For this review, take the finished solid that the model builds, in its own axes (mm). A direction names the side the tool comes from. Coordinates: 2 decimals unless noted, no trailing zeros. Order: outer loops, then holes, each group sorted by start corner. A loop starts at its lowest first (then second) coordinate and runs counter-clockwise, first axis right, second up.
from build123d import *

# Parameters (mm, degrees)
F1_DEPTH = 25
F2_R     = 8
F3_DEPTH = 37.501


with BuildPart() as f1:
    # F0 (on Front) → F1 (new body)
    with BuildSketch(Plane.XZ):
        with BuildLine():
            Line((-51.7705098312, 2.5), (-22.360679775, 2.5))
            ThreePointArc((-22.360679775, 2.5), (-20.5395959064, 9.1855865354), (-16.7705098312, 15))
            Line((-16.7705098312, 15), (-51.7705098312, 15))
            Line((-51.7705098312, 15), (-51.7705098312, 2.5))
        make_face()
        with BuildLine():
            ThreePointArc((-16.7705098312, -15), (-20.5395959064, -9.1855865354), (-22.360679775, -2.5))
            Line((-22.360679775, -2.5), (-51.7705098312, -2.5))
            Line((-51.7705098312, -2.5), (-51.7705098312, -15))
            Line((-51.7705098312, -15), (-16.7705098312, -15))
        make_face()
        with BuildLine():
            ThreePointArc((-14.7901994577, 2.5), (1.2543939042, 14.9474578418), (15, 0))
            ThreePointArc((15, 0), (1.2543939042, -14.9474578418), (-14.7901994577, -2.5))
            Line((-14.7901994577, -2.5), (-22.360679775, -2.5))
            ThreePointArc((-22.360679775, -2.5), (-20.5395959064, -9.1855865354), (-16.7705098312, -15))
            ThreePointArc((-16.7705098312, -15), (8.0284970199, -21.0188780767), (22.5, 0))
            ThreePointArc((22.5, 0), (8.0284970199, 21.0188780767), (-16.7705098312, 15))
            ThreePointArc((-16.7705098312, 15), (-20.5395959064, 9.1855865354), (-22.360679775, 2.5))
            Line((-22.360679775, 2.5), (-14.7901994577, 2.5))
        make_face()
    extrude(amount=F1_DEPTH)

    # F2 (on face) → F3 (cut, through all)
    with BuildSketch(Plane.XY.offset(15)):
        with Locations((-34.2705098312, -12.5)):
            Circle(F2_R)
    extrude(amount=-F3_DEPTH, mode=Mode.SUBTRACT)


solid = f1.part
1. Take a section at D-D, the plane y = -22.5. Give the boundary of the cut face in (x, z).
Answer below:
outline: (-51.77, -15) - (-16.77, -15) arc R22.5 ccw (long way) to (-16.77, 15) - (-51.77, 15) - (-51.77, 2.5) - (-14.79, 2.5) arc R15 cw (long way) to (-14.79, -2.5) - (-51.77, -2.5) - close
2. Machinability: for faces 4 (the face through (-15, 0, -5)), 5 (the face through (-25, -12, -2.5)), 6 (the face through (-26, -12, 15)), 7 (the face through (-42.3, -9.5, -15)), which of the approach directions +Z, -Z, +X, -X, +Y, -Y give a long, thin tool a straight path to every point of the face, cutting with its end or side? Answer none if there is none.
Answer below:
face 4: +Z, -Z, +X, -X, +Y
face 5: -X, +Y, -Y
face 6: +Z, -X, +Y, -Y
face 7: -Z, -X, +Y, -Y
3. Clearance check with flat-ended pins moving along their axes: pin 1 Ø14.5 at (x, y) = (-34.27, -12.5) entering from -Z; pin 2 Ø8 at (x, y) = (-23, -8) entering from +Z; pin 3 Ø10 at (x, y) = (-42.5, -8.5) entering from -Z; pin 4 Ø2 at (y, z) = (-10.5, 17.5) entering from -X. State where each tip first meets the part, or that it passes through.
Answer below:
pin 1: passes through
pin 2: stops at z = 15
pin 3: stops at z = -15
pin 4: stops at x = -15.3
4. To check wall thickness, follow L1, parallel to Z at x = 0, y = -13.25; L2, parallel to Z at x = -45, y = -4.5; L3, parallel to X at y = -6, z = -10.5. State the ranges of each line that lie inside material, in increasing order.
Answer below:
L1: z = -22.5 to -15, 15 to 22.5
L2: z = -15 to -2.5, 2.5 to 15
L3: x = -51.77 to -38.93, -29.61 to -10.71, 10.71 to 19.9
5. Take a section at A-A, the plane z = -4. Give the boundary of the cut face in (x, y), plus the area to 3 significant figures.
Answer below:
outline: (-51.77, -25) - (-14.46, -25) - (-14.46, 0) - (-51.77, 0) - close; (14.46, -25) - (22.14, -25) - (22.14, 0) - (14.46, 0) - close; hole circle Ø16 at (-34.27, -12.5)
area: 924 mm2
6. Take a section at C-C, the plane y = -16.75. Give the boundary of the cut face in (x, z).
Answer below:
outline: (-51.77, -15) - (-41.05, -15) - (-41.05, -2.5) - (-51.77, -2.5) - close; (-51.77, 2.5) - (-41.05, 2.5) - (-41.05, 15) - (-51.77, 15) - close; (-27.49, -15) - (-16.77, -15) arc R22.5 ccw (long way) to (-16.77, 15) - (-27.49, 15) - (-27.49, 2.5) - (-14.79, 2.5) arc R15 cw (long way) to (-14.79, -2.5) - (-27.49, -2.5) - close
7. The part is to be moulded in two halves that separate along X. For faces 1 (the face through (14.987, -12.325, 0.624)), 2 (the face through (-51.771, -12, -9)), 3 (the face through (-25, -12, 2.5)), say which applies: +X half, -X half, draft (parallel to the pull), parting line (faces both ways), or undercut.
Answer below:
face 1: undercut
face 2: -X half
face 3: draft
8. Take a section at B-B, the plane x = 0. Give the boundary of the cut face in (y, z).
Answer below:
outline: (-25, -22.5) - (0, -22.5) - (0, -15) - (-25, -15) - close; (-25, 15) - (0, 15) - (0, 22.5) - (-25, 22.5) - close
